from build123d import *

# Parameters (mm, degrees)
F0_W      = 69.24
F0_H      = 17
F0_R      = 1.25
F0_W_2    = 15
F0_H_2    = 10
F1_DEPTH  = 5
F2_R      = 0.8
F2_W      = 19.22
F2_H      = 4
F3_DEPTH  = 25
F4_R      = 1.25
F5_DEPTH  = 25
F6_R      = 3
F7_DEPTH  = 17
F8_R      = 1.25
F9_DEPTH  = 25
F10_R     = 3
F11_DEPTH = 17
F12_W     = 20
F12_H     = 17
F13_DEPTH = 2


with BuildPart() as f1:
    # F0 (on Top) → F1 (new body, symmetric)
    with BuildSketch(Plane.XY):
        Rectangle(F0_W, F0_H)
        with Locations((-26, 0)):
            Circle(F0_R, mode=Mode.SUBTRACT)
        Rectangle(F0_W_2, F0_H_2, mode=Mode.SUBTRACT)
        with Locations((26, 0)):
            Circle(F0_R, mode=Mode.SUBTRACT)
    extrude(amount=F1_DEPTH, both=True)

    # F2 (on face) → F3 (cut)
    with BuildSketch(Plane.XZ.offset(8.5)):
        Circle(F2_R)
        with Locations((-25.01, 0)):
            Rectangle(F2_W, F2_H)
        with Locations((25.01, 0)):
            Rectangle(F2_W, F2_H)
    extrude(amount=-F3_DEPTH, mode=Mode.SUBTRACT)

    # F4 (on face) → F5 (cut)
    with BuildSketch(Plane(origin=(-34.62, 0, 0), x_dir=(0, -1, 0), z_dir=(-1, 0, 0))):
        Circle(F4_R)
    extrude(amount=-F5_DEPTH, mode=Mode.SUBTRACT)

    # F6 (on face) → F7 (cut)
    with BuildSketch(Plane(origin=(-34.62, 0, 0), x_dir=(0, -1, 0), z_dir=(-1, 0, 0))):
        Circle(F6_R)
    extrude(amount=-F7_DEPTH, mode=Mode.SUBTRACT)

    # F8 (on face) → F9 (cut)
    with BuildSketch(Plane.YZ.offset(34.62)):
        Circle(F8_R)
    extrude(amount=-F9_DEPTH, mode=Mode.SUBTRACT)

    # F10 (on face) → F11 (cut)
    with BuildSketch(Plane.YZ.offset(34.62)):
        Circle(F10_R)
    extrude(amount=-F11_DEPTH, mode=Mode.SUBTRACT)

    # F12 (on face) → F13 (cut)
    with BuildSketch(Plane.XY.offset(5)):
        Rectangle(F12_W, F12_H)
    extrude(amount=-F13_DEPTH, mode=Mode.SUBTRACT)


solid = f1.part
Design review of the part built by this model. Coordinates are the model's own, in mm. A direction names the side the tool comes from. Coordinates: 2 decimals unless noted, no trailing zeros. Loops run counter-clockwise (first coordinate to the right, second up) from the corner with the lowest first, then second, coordinate; pieces in that order, holes last. Notation, with made-up numbers: (61.25, -7.75) -> (78.25, -7.75) arc R25 cw to (78.25, 16.25) -> close; hole circle Ø8 at (58, 27.25). An arc over 180 degrees is marked (long way). Use a Markdown table: item, result. Add a question column.
Item 1: The part is to be moulded in two halves that separate along Y. For faces 5 (the flat face through (-25, -4, -2)), 6 (the flat face through (0, 5, -1)), 7 (the flat face through (0, 8.5, -1)), say which applies: +Y half, -Y half, draft (parallel to the pull), parting line (faces both ways), or undercut.
Item 2: Wall thickness on L1, parallel to Z at x = 23, y = 5.5; L2, parallel to Y at x = 7, z = -3.75; L3, parallel to X at y = 0, z = 4.55: over which ranges is each line inside the solid? List them lowest first. Write a range as from..to.
Item 3: We need section A-A, the plane x = -26. Write out the cut boundary in (y, z), and give its area (3 significant figures).
Item 4: Machinability: for faces 1 (the flat face through (-10, 0, 4)), 2 (the cylindrical face through (26.239, 1.565, -2.559)), 3 (the flat face through (25, -4, 2)), 4 (the cylindrical face through (-12.55, 0.27, -1.22)), which of the approach directions +Z, -Z, +X, -X, +Y, -Y give a long, thin tool a straight path to every point of the face, cutting with its end or side? Answer none if there is none.
Item 5: We need section C-C, the plane x = -18.5. Write out the cut boundary in (y, z), and give its area (3 significant figures).
Item 6: We need section D-D, the plane z = 0. Write out the cut boundary in (x, y).
Item 7: We need section B-B, the plane y = 7. Write out the cut boundary in (x, z).
Item 8: Clearance check with flat-ended pins moving along their axes: P1, Ø2, axis at y = 0, z = 0, coming from the -X side; P2, Ø2, axis at y = 1, z = -0.5, coming from the +X side; P3, Ø1.2, axis at y = 0.5, z = 0, coming from the +X side; P4, Ø2, axis at x = 0, z = 0, coming from the -Y side. State where each tip first meets the part, or that it passes through.
Numbers:
| question | item | result |
|---|---|---|
| 1 | face 5 | draft |
| 1 | face 6 | undercut |
| 1 | face 7 | +Y half |
| 2 | L1 | z = -5..-2, 2..5 |
| 2 | L2 | y = -8.5..-5, 5..8.5 |
| 2 | L3 | x = -34.62..-27.25, -24.75..-10, 10..24.75, 27.25..34.62 |
| 3 | outline | (-8.5, -5) -> (-1.25, -5) -> (-1.25, -2.73) arc R3 cw to (-2.24, -2) -> (-8.5, -2) -> close; (-8.5, 2) -> (-2.24, 2) arc R3 cw to (-1.25, 2.73) -> (-1.25, 5) -> (-8.5, 5) -> close; (1.25, -5) -> (8.5, -5) -> (8.5, -2) -> (2.24, -2) arc R3 cw to (1.25, -2.73) -> close; (1.25, 2.73) arc R3 cw to (2.24, 2) -> (8.5, 2) -> (8.5, 5) -> (1.25, 5) -> close |
| 3 | area | 85.4 mm^2 |
| 4 | face 1 | +Z, +Y, -Y |
| 4 | face 2 | +X |
| 4 | face 3 | +X, +Y, -Y |
| 4 | face 4 | -X |
| 5 | outline | (-8.5, -5) -> (8.5, -5) -> (8.5, -2) -> (2.24, -2) arc R3 cw to (-2.24, -2) -> (-8.5, -2) -> close; (-8.5, 2) -> (-2.24, 2) arc R3 cw to (2.24, 2) -> (8.5, 2) -> (8.5, 5) -> (-8.5, 5) -> close |
| 5 | area | 95.8 mm^2 |
| 6 | outline | (-15.4, -8.5) -> (-0.8, -8.5) -> (-0.8, -5) -> (-7.5, -5) -> (-7.5, 5) -> (-0.8, 5) -> (-0.8, 8.5) -> (-15.4, 8.5) -> (-15.4, 1.25) -> (-9.62, 1.25) -> (-9.62, -1.25) -> (-15.4, -1.25) -> close; (0.8, -8.5) -> (15.4, -8.5) -> (15.4, -1.25) -> (9.62, -1.25) -> (9.62, 1.25) -> (15.4, 1.25) -> (15.4, 8.5) -> (0.8, 8.5) -> (0.8, 5) -> (7.5, 5) -> (7.5, -5) -> (0.8, -5) -> close |
| 7 | outline | (-34.62, -5) -> (34.62, -5) -> (34.62, -2) -> (15.4, -2) -> (15.4, 2) -> (34.62, 2) -> (34.62, 5) -> (10, 5) -> (10, 3) -> (-10, 3) -> (-10, 5) -> (-34.62, 5) -> (-34.62, 2) -> (-15.4, 2) -> (-15.4, -2) -> (-34.62, -2) -> close; hole circle Ø1.6 at (0, 0) |
| 8 | P1 | stops at x = -9.62 |
| 8 | P2 | stops at x = 15.4 |
| 8 | P3 | stops at x = 9.62 |
| 8 | P4 | stops at y = -8.5 |
